Input: part model. Units: mm. Frame: model coordinates. A direction names the side the tool comes from. Round coordinates to 2 decimals unless told otherwise and drop trailing zeros. Loops run counter-clockwise (first coordinate to the right, second up) from the corner with the lowest first, then second, coordinate; pieces in that order, holes last. Notation, with made-up numbers: (-35.75, 0.5) -> (-18.75, 0.5) arc R16 ccw to (-18.75, 28.5) -> close; hole circle Ø3 at (43.25, 28.5). An arc over 180 degrees is marked (long way). Answer in a Markdown table with one row per item. Add a question column.
Q1. Ray query, L1, parallel to Z at x = 95, y = -3.2; L2, parallel to X at y = -1.45, z = -45; L3, parallel to X at y = -4, z = -12. Return the intervals inside material, ascending. Write a range as from..to.
Q2. Pin query (flat end, axial travel): pin 1 (2.5 mm diameter, centred on y = -1.5, z = -45.5, fed in from -X). Return the tip coordinate at first contact, or that it passes through.
Q3. Section B-B, the plane z = -45. Output: boundary loops of the cut face in (x, y).
Q4. Section D-D, the plane z = -2. Output: boundary loops of the cut face in (x, y), and give its area (3 significant figures).
Q5. Mould query, pull axis Z, two halves, no side actions, for faces 4 (the face through (-115, -2, 0)), 5 (the face through (84, -2, 42.5)), 6 (the face through (-92, -2, -42.5)). Classes: pulls with the +Z half, pulls with the -Z half, needs draft (parallel to the pull), parting line crosses it, or undercut.
Q6. Section C-C, the plane x = 95. Output: boundary loops of the cut face in (y, z).
Q7. Section A-A, the plane x = 0. Output: boundary loops of the cut face in (y, z), and give its area (3 significant figures).
Q8. Reachability of faces 1 (the face through (46, -2, 33)), 2 (the face through (-112, -2, -25.5)), 3 (the face through (23, -2, -45)) from +Z, -Z, +X, -X, +Y, -Y: full face, straight path, thin tool, end or side. Return the list, or none.
```python
from build123d import *

# Parameters (mm, degrees)
F0_W     = 46
F0_H     = 5
F0_W_2   = 5
F0_H_2   = 17
F0_R     = 2.75
F1_DEPTH = 5


with BuildPart() as f1:
    # F0 (on Front) → F1 (new body)
    with BuildSketch(Plane.XZ):
        with BuildLine():
            Line((115, 42.5), (110, 42.5))
            Line((110, 42.5), (46, 42.5))
            Line((46, 42.5), (46, 23.5))
            ThreePointArc((46, 23.5), (0, -22.5), (-46, 23.5))
            Line((-46, 23.5), (-46, 42.5))
            Line((-46, 42.5), (-110, 42.5))
            Line((-110, 42.5), (-115, 42.5))
            Line((-115, 42.5), (-115, 25.5))
            Line((-115, 25.5), (-110, 25.5))
            Line((-110, 25.5), (-110, 8.5))
            Line((-110, 8.5), (-115, 8.5))
            Line((-115, 8.5), (-115, -8.5))
            Line((-115, -8.5), (-110, -8.5))
            Line((-110, -8.5), (-110, -25.5))
            Line((-110, -25.5), (-115, -25.5))
            Line((-115, -25.5), (-115, -42.5))
            Line((-115, -42.5), (-69, -42.5))
            Line((-69, -42.5), (-69, -47.5))
            Line((-69, -47.5), (-115, -47.5))
            Line((-115, -47.5), (-115, -52.5))
            Line((-115, -52.5), (115, -52.5))
            Line((115, -52.5), (120, -52.5))
            Line((120, -52.5), (120, 42.5))
            Line((120, 42.5), (115, 42.5))
        make_face()
        with Locations((0, -45)):
            Rectangle(F0_W, F0_H, mode=Mode.SUBTRACT)
        with Locations((92, -45)):
            Rectangle(F0_W, F0_H, mode=Mode.SUBTRACT)
        with Locations((112.5, -17)):
            Rectangle(F0_W_2, F0_H_2, mode=Mode.SUBTRACT)
        with Locations((112.5, 17)):
            Rectangle(F0_W_2, F0_H_2, mode=Mode.SUBTRACT)
        with Locations((95, 22.5)):
            Circle(F0_R, mode=Mode.SUBTRACT)
    extrude(amount=F1_DEPTH)


solid = f1.part
```
Answer block:
| question | item | result |
|---|---|---|
| 1 | L1 | -52.5..-47.5, -42.5..19.75, 25.25..42.5 |
| 1 | L2 | -69..-23, 23..69, 115..120 |
| 1 | L3 | -110..-29.25, 29.25..110, 115..120 |
| 2 | pin 1 | x = -69 |
| 3 | outline | (-69, -5) -> (-23, -5) -> (-23, 0) -> (-69, 0) -> close; (23, -5) -> (69, -5) -> (69, 0) -> (23, 0) -> close; (115, -5) -> (120, -5) -> (120, 0) -> (115, 0) -> close |
| 4 | outline | (-115, -5) -> (-38.29, -5) -> (-38.29, 0) -> (-115, 0) -> close; (38.29, -5) -> (120, -5) -> (120, 0) -> (38.29, 0) -> close |
| 4 | area | 792 mm^2 |
| 5 | face 4 | needs draft |
| 5 | face 5 | pulls with the +Z half |
| 5 | face 6 | undercut |
| 6 | outline | (-5, -52.5) -> (0, -52.5) -> (0, -47.5) -> (-5, -47.5) -> close; (-5, -42.5) -> (0, -42.5) -> (0, 19.75) -> (-5, 19.75) -> close; (-5, 25.25) -> (0, 25.25) -> (0, 42.5) -> (-5, 42.5) -> close |
| 7 | outline | (-5, -52.5) -> (0, -52.5) -> (0, -47.5) -> (-5, -47.5) -> close; (-5, -42.5) -> (0, -42.5) -> (0, -22.5) -> (-5, -22.5) -> close |
| 7 | area | 125 mm^2 |
| 8 | face 1 | +Z, +Y, -Y |
| 8 | face 2 | -X, +Y, -Y |
| 8 | face 3 | +Y, -Y |
